Read the model definition and answer for the solid it produces. Units are mm, in the model's axes. A direction names the side the tool comes from. Give positions to 0.01 mm unless a question says otherwise; leave off trailing zeros. Order: outer loops, then holes, each group sorted by start corner. A loop starts at its lowest first (then second) coordinate and runs counter-clockwise, first axis right, second up.
```python
from build123d import *

# Parameters (mm, degrees)
ESBO_O1_W                = 74
ESBO_O1_H                = 40
RESSALTO_EXTRUS_O1_DEPTH = 3
ESBO_O2_W                = 22
ESBO_O2_H                = 3
ESBO_O2_W_2              = 3
ESBO_O2_H_2              = 20
CORTE_EXTRUS_O1_DEPTH    = 3
ESBO_O3_R                = 3.25
CORTE_EXTRUS_O2_DEPTH    = 10


with BuildPart() as part:
    # Esboço1 → Ressalto-extrusão1 (new body)
    with BuildSketch(Plane.XY):
        Rectangle(ESBO_O1_W, ESBO_O1_H)
    extrude(amount=RESSALTO_EXTRUS_O1_DEPTH)

    # Esboço2 → Corte-extrusão1 (cut)
    with BuildSketch(Plane.XY.offset(3)):
        with Locations((-26, -18.5)):
            Rectangle(ESBO_O2_W, ESBO_O2_H)
        with Locations((26, -18.5)):
            Rectangle(ESBO_O2_W, ESBO_O2_H)
        with Locations((-35.5, 0)):
            Rectangle(ESBO_O2_W_2, ESBO_O2_H_2)
        with Locations((35.5, 0)):
            Rectangle(ESBO_O2_W_2, ESBO_O2_H_2)
    extrude(amount=-CORTE_EXTRUS_O1_DEPTH, mode=Mode.SUBTRACT)

    # Esboço3 → Corte-extrusão2 (cut)
    with BuildSketch(Plane.XY.offset(3)):
        with Locations((-23, -7)):
            Circle(ESBO_O3_R)
    extrude(amount=-CORTE_EXTRUS_O2_DEPTH, mode=Mode.SUBTRACT)


solid = part.part
```
1) The part is cut by section D-D on x = 19. Determine the outline of the cut face in (y, z), and give its area (3 significant figures).
Final values:
outline: (-17, 0) - (20, 0) - (20, 3) - (-17, 3) - close
area: 111 mm2
2) Given pin 1 (0.9 mm diameter, centred on x = -36, z = 1, fed in from -Y); pin 2 (1.5 mm diameter, centred on y = -1.5, z = 1, fed in from -X); pin 3 (0.9 mm diameter, centred on y = -18, z = 1.5, fed in from -X), each flat-ended and moving along its own axis, determine where each tip first touches the part or whether it passes through.
Final values:
pin 1: stops at y = -17
pin 2: stops at x = -34
pin 3: stops at x = -15
3) The part is cut by section A-A on y = -7. Determine the outline of the cut face in (x, z).
Final values:
outline: (-34, 0) - (-26.25, 0) - (-26.25, 3) - (-34, 3) - close; (-19.75, 0) - (34, 0) - (34, 3) - (-19.75, 3) - close
4) The part is cut by section B-B on z = 0.95. Determine the outline of the cut face in (x, y).
Final values:
outline: (-37, -17) - (-15, -17) - (-15, -20) - (15, -20) - (15, -17) - (37, -17) - (37, -10) - (34, -10) - (34, 10) - (37, 10) - (37, 20) - (-37, 20) - (-37, 10) - (-34, 10) - (-34, -10) - (-37, -10) - close; hole circle Ø6.5 at (-23, -7)
5) For a pull along X with two mould halves and no side action, classify faces 4 (the face through (-26, -17, 2)), 5 (the face through (37, -14, 1)), 6 (the face through (-37, -14, 1)), 7 (the face through (-26.247, -6.857, 1.521)) as released by +X, released by -X, zero draft, split by the parting line, or undercut.
Final values:
face 4: zero draft
face 5: released by +X
face 6: released by -X
face 7: undercut
6) A tool of negligible diameter and unlimited length cuts with its end or side. For faces 1 (the face through (26, -17, 2)), 2 (the face through (-36, -10, 2)), 3 (the face through (35, 10, 2)), from which of +Z, -Z, +X, -X, +Y, -Y can it reach the whole face along a straight path? Write none if from no direction.
Final values:
face 1: +Z, -Z, +X, -Y
face 2: +Z, -Z, -X
face 3: +Z, -Z, +X
7) The part is cut by section C-C on x = -23. Determine the outline of the cut face in (y, z).
Final values:
outline: (-17, 0) - (-10.25, 0) - (-10.25, 3) - (-17, 3) - close; (-3.75, 0) - (20, 0) - (20, 3) - (-3.75, 3) - close
8) Consider L1, parallel to Y at x = -23, z = 1.5; L2, parallel to Y at x = 33.5, z = 2.2; L3, parallel to X at y = -3, z = 1.15. Determine where each line is inside the solid, lowest interval first.
Final values:
L1: y = -17 to -10.25, -3.75 to 20
L2: y = -17 to 20
L3: x = -34 to 34
